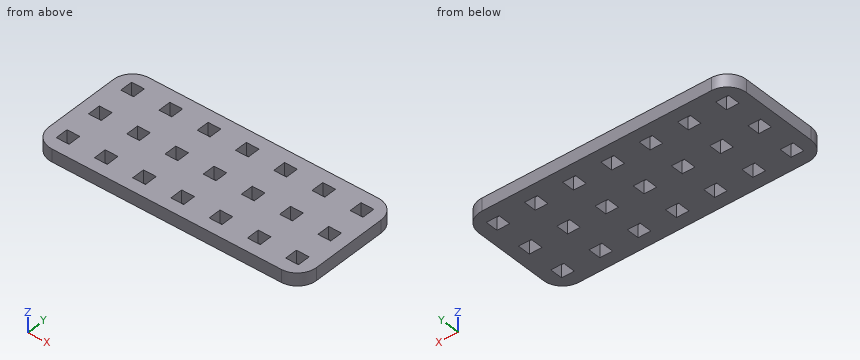
from build123d import *

# Parameters (mm, degrees)
MODEL_W                 = 3
MODEL_H                 = 3
SALIENTE_EXTRUIR1_DEPTH = 3


with BuildPart() as part:
    # Model → Saliente-Extruir1 (new body)
    with BuildSketch(Plane.XY):
        with BuildLine():
            Line((13.663940534, 300.565078072), (67.663940534, 300.565078072))
            ThreePointArc((67.663940534, 300.565078072), (70.845921049, 299.247058587), (72.163940534, 296.065078072))
            Line((72.163940534, 296.065078072), (72.163940534, 278.065078072))
            ThreePointArc((72.163940534, 278.065078072), (70.845921049, 274.883097556), (67.663940534, 273.565078072))
            Line((67.663940534, 273.565078072), (13.663940534, 273.565078072))
            ThreePointArc((13.663940534, 273.565078072), (10.481960019, 274.883097556), (9.163940534, 278.065078072))
            Line((9.163940534, 278.065078072), (9.163940534, 296.065078072))
            ThreePointArc((9.163940534, 296.065078072), (10.481960019, 299.247058587), (13.663940534, 300.565078072))
        make_face()
        with Locations((13.663940534, 296.065078072)):
            Rectangle(MODEL_W, MODEL_H, mode=Mode.SUBTRACT)
        with Locations((22.663940534, 296.065078072)):
            Rectangle(MODEL_W, MODEL_H, mode=Mode.SUBTRACT)
        with Locations((31.663940534, 296.065078072)):
            Rectangle(MODEL_W, MODEL_H, mode=Mode.SUBTRACT)
        with Locations((58.663940534, 296.065078072)):
            Rectangle(MODEL_W, MODEL_H, mode=Mode.SUBTRACT)
        with Locations((67.663940534, 296.065078072)):
            Rectangle(MODEL_W, MODEL_H, mode=Mode.SUBTRACT)
        with Locations((13.663940534, 278.065078072)):
            Rectangle(MODEL_W, MODEL_H, mode=Mode.SUBTRACT)
        with Locations((22.663940534, 278.065078072)):
            Rectangle(MODEL_W, MODEL_H, mode=Mode.SUBTRACT)
        with Locations((31.663940534, 278.065078072)):
            Rectangle(MODEL_W, MODEL_H, mode=Mode.SUBTRACT)
        with Locations((58.663940534, 278.065078072)):
            Rectangle(MODEL_W, MODEL_H, mode=Mode.SUBTRACT)
        with Locations((67.663940534, 278.065078072)):
            Rectangle(MODEL_W, MODEL_H, mode=Mode.SUBTRACT)
        with Locations((13.663940534, 287.065078072)):
            Rectangle(MODEL_W, MODEL_H, mode=Mode.SUBTRACT)
        with Locations((22.663940534, 287.065078072)):
            Rectangle(MODEL_W, MODEL_H, mode=Mode.SUBTRACT)
        with Locations((31.663940534, 287.065078072)):
            Rectangle(MODEL_W, MODEL_H, mode=Mode.SUBTRACT)
        with Locations((58.663940534, 287.065078072)):
            Rectangle(MODEL_W, MODEL_H, mode=Mode.SUBTRACT)
        with Locations((67.663940534, 287.065078072)):
            Rectangle(MODEL_W, MODEL_H, mode=Mode.SUBTRACT)
        with Locations((40.663940534, 296.065078072)):
            Rectangle(MODEL_W, MODEL_H, mode=Mode.SUBTRACT)
        with Locations((49.663940534, 296.065078072)):
            Rectangle(MODEL_W, MODEL_H, mode=Mode.SUBTRACT)
        with Locations((40.663940534, 278.065078072)):
            Rectangle(MODEL_W, MODEL_H, mode=Mode.SUBTRACT)
        with Locations((49.663940534, 278.065078072)):
            Rectangle(MODEL_W, MODEL_H, mode=Mode.SUBTRACT)
        with Locations((40.663940534, 287.065078072)):
            Rectangle(MODEL_W, MODEL_H, mode=Mode.SUBTRACT)
        with Locations((49.663940534, 287.065078072)):
            Rectangle(MODEL_W, MODEL_H, mode=Mode.SUBTRACT)
    extrude(amount=SALIENTE_EXTRUIR1_DEPTH)


solid = part.part
Source: CAD feature listing. Evaluate the final solid. Frame: model axes, mm. Give positions to 0.01 mm unless a question says otherwise; leave off trailing zeros. Order: outer loops, then holes, each group sorted by start corner. A loop starts at its lowest first (then second) coordinate and runs counter-clockwise, first axis right, second up. Notation, with made-up numbers: (-14, 62) -> (6, 62) arc R9 cw to (6, 66) -> close; hole circle Ø5 at (73, 0.25). An arc over 180 degrees is marked (long way). Use a Markdown table: item, result.
1) Section query A-A, the plane x = 49.5. Return the cut outline in (y, z), then the cut area to 3 significant figures.
Answer list:
| item | result |
|---|---|
| outline | (273.57, 0) -> (276.57, 0) -> (276.57, 3) -> (273.57, 3) -> close; (279.57, 0) -> (285.57, 0) -> (285.57, 3) -> (279.57, 3) -> close; (288.57, 0) -> (294.57, 0) -> (294.57, 3) -> (288.57, 3) -> close; (297.57, 0) -> (300.57, 0) -> (300.57, 3) -> (297.57, 3) -> close |
| area | 54.0 mm² |
2) Contact query for a flat-ended pin moving along its axis: P1, Ø1.5, axis at x = 13.5, z = 1, coming from the +Y side. Output: stop coordinate, or through.
Answer list:
| item | result |
|---|---|
| P1 | y = 300.57 |
3) Section query C-C, the plane y = 298.25. Return the cut outline in (x, z), then the cut area to 3 significant figures.
Answer list:
| item | result |
|---|---|
| outline | (9.73, 0) -> (71.6, 0) -> (71.6, 3) -> (9.73, 3) -> close |
| area | 186 mm² |
4) Section query B-B, the plane z = 1.6. Count the separate pieces of the cut face and the enclosed holes in it, then the cut area to 3 significant figures.
Answer list:
| item | result |
|---|---|
| separate pieces | 1 |
| enclosed holes | 21 |
| area | 1,490 mm² |
5) Ray query, line 1 along Y through (x, z) = (40.5, 2.55); line 2 along X through (y, z) = (298, 1.35); line 3 along X through (y, z) = (275.5, 1.75). Return the intervals inside material, ascending. Write a range as [from, to].
Answer list:
| item | result |
|---|---|
| line 1 | [273.57, 276.57], [279.57, 285.57], [288.57, 294.57], [297.57, 300.57] |
| line 2 | [9.6, 71.73] |
| line 3 | [9.97, 71.36] |
